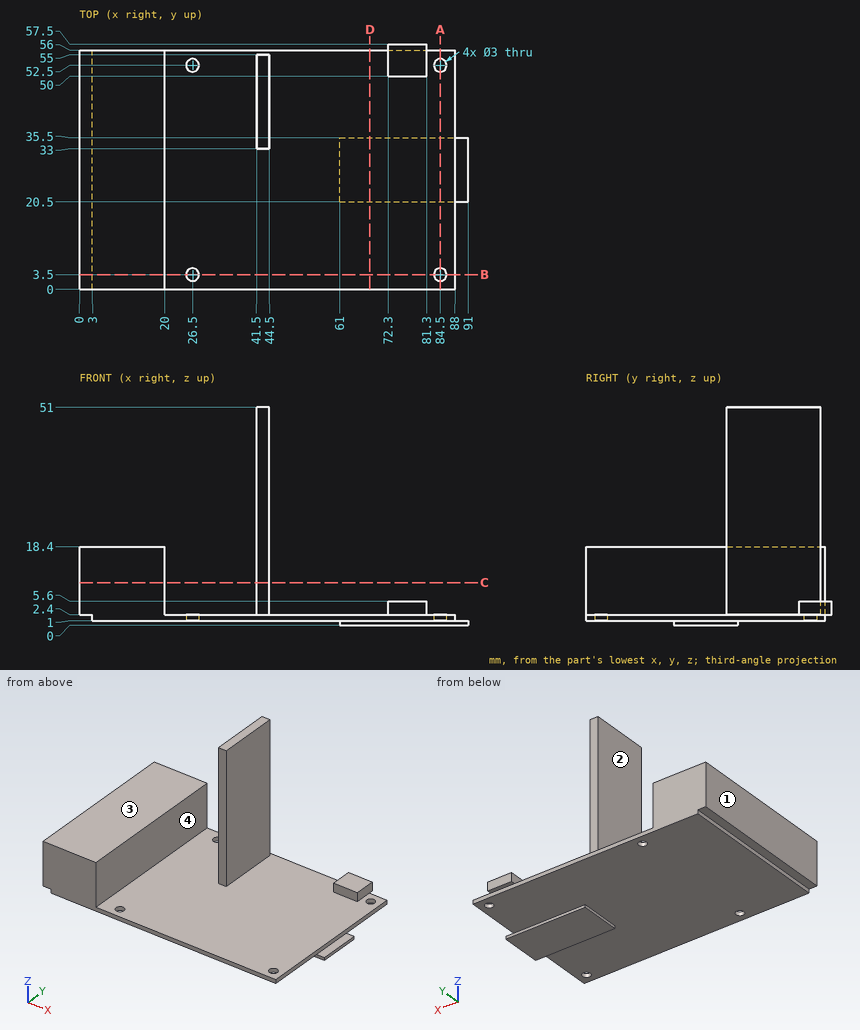
Can you work these out from the drawing? Everything is in mm from the part's minimum corner. Coordinates: 2 decimals unless noted, no trailing zeros. Order: outer loops, then holes, each group sorted by start corner. A loop starts at its lowest first (then second) coordinate and runs counter-clockwise, first axis right, second up. Notation, with made-up numbers: (-20.5, 78.25) -> (32.5, 78.25) arc R27 cw to (32.5, 117.25) -> close; hole circle Ø3 at (-38, 63). An arc over 180 degrees is marked (long way). Return JSON: item names as keys, results as strings.
1) I'm going to push flat-ended pins straight in: P1, Ø17, axis at x = 67.5, y = 29, coming from the +Z side; P2, Ø3.5, axis at x = 26.5, y = 3.5, coming from the -Z side; P3, Ø0.7, axis at y = 19, z = 2, coming from the +X side. Where does each tip first touch, or does it pass through?
Conclusion:
{"P1": "stops at z = 2.4", "P2": "stops at z = 1", "P3": "stops at x = 88"}
2) If we section it at A-A on x = 84.5: List the corners of the cut face in (y, z) for me, plus the area to 3 significant figures.
Conclusion:
{"outline": "(0, 1) -> (2, 1) -> (2, 2.4) -> (0, 2.4) -> close; (5, 1) -> (20.5, 1) -> (20.5, 0) -> (35.5, 0) -> (35.5, 1) -> (51, 1) -> (51, 2.4) -> (5, 2.4) -> close; (54, 1) -> (56, 1) -> (56, 2.4) -> (54, 2.4) -> close", "area": "85.0 mm²"}
3) If we section it at D-D on x = 68: List the corners of the cut face in (y, z) for me.
Conclusion:
{"outline": "(0, 1) -> (20.5, 1) -> (20.5, 0) -> (35.5, 0) -> (35.5, 1) -> (56, 1) -> (56, 2.4) -> (0, 2.4) -> close"}
4) If we section it at B-B on y = 3.5: List the corners of the cut face in (x, z) for me, plus the area to 3 significant figures.
Conclusion:
{"outline": "(0, 2.4) -> (3, 2.4) -> (3, 1) -> (25, 1) -> (25, 2.4) -> (20, 2.4) -> (20, 18.4) -> (0, 18.4) -> close; (28, 1) -> (83, 1) -> (83, 2.4) -> (28, 2.4) -> close; (86, 1) -> (88, 1) -> (88, 2.4) -> (86, 2.4) -> close", "area": "431 mm²"}
5) If I drill on probe 1 along Y at (x, z) = (84.5, 1.9); probe 2 along X at (y, z) = (35, 3); probe 3 along X at (y, z) = (35, 20), over which ranges is the centre line in solid material (lowest first)?
Conclusion:
{"probe 1": "y = 0 to 2, 5 to 51, 54 to 56", "probe 2": "x = 0 to 20, 41.5 to 44.5", "probe 3": "x = 41.5 to 44.5"}
6) If we section it at C-C on z = 10: List the corners of the cut face in (x, y) for me.
Conclusion:
{"outline": "(0, 0) -> (20, 0) -> (20, 56) -> (0, 56) -> close; (41.5, 33) -> (44.5, 33) -> (44.5, 55) -> (41.5, 55) -> close"}
7) Thinking about a two-plate mould opening in X: for the marked faces 1, 2, 3 and 4, which applies, +X half, -X half, draft (parallel to the pull), parting line (faces both ways), or undercut?
Conclusion:
{"face 1": "-X half", "face 2": "undercut", "face 3": "draft", "face 4": "undercut"}
